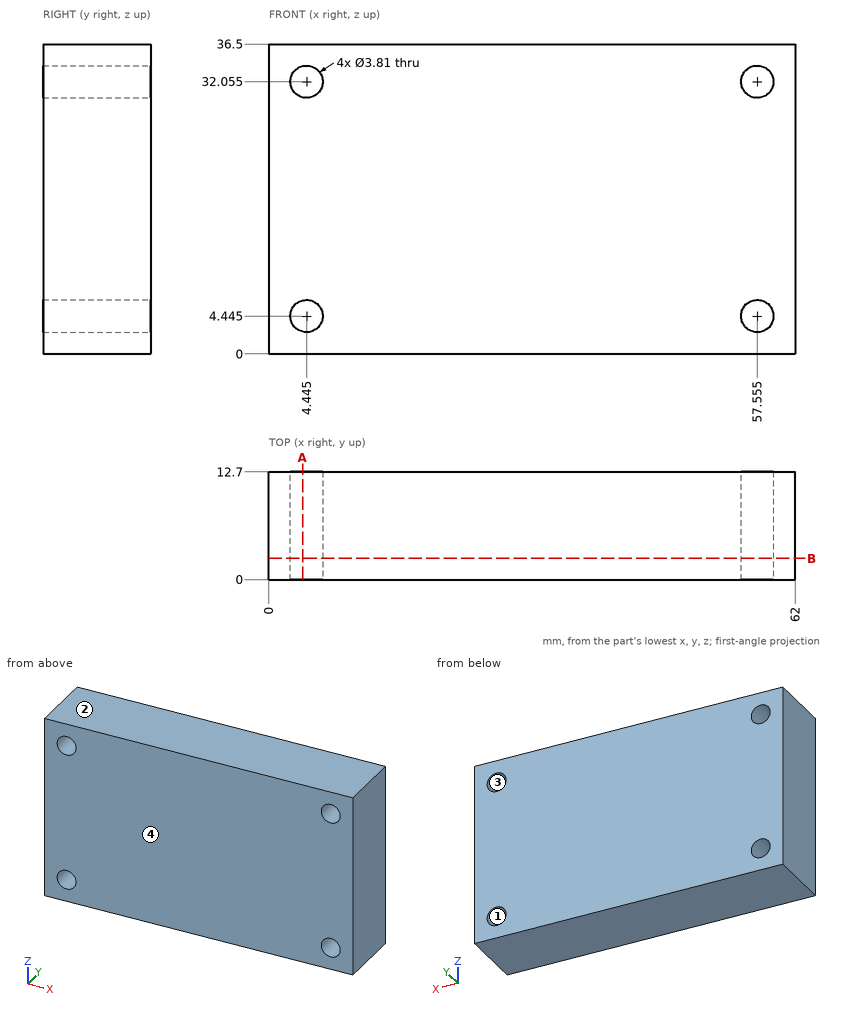
Source: three-view drawing plus pictorial views. Frame: mm from the lowest corner of the part. Coordinates: 2 decimals unless noted, no trailing zeros. Loops run counter-clockwise (first coordinate to the right, second up) from the corner with the lowest first, then second, coordinate; pieces in that order, holes last. Notation, with made-up numbers: (65.25, 46) -> (107.25, 46) arc R23 cw to (107.25, 85) -> close; hole circle Ø11 at (18.25, 52.5). An arc over 180 degrees is marked (long way). One line per item, written item: value.
(1) Cut plane B-B (y = 2.5). Output: boundary loops of the cut face in (x, z) (3 decimals), then the cut area to 3 significant figures.
Answer below:
outline: (0, 0) -> (62, 0) -> (62, 36.5) -> (0, 36.5) -> close; hole circle Ø3.81 at (4.445, 4.445); hole circle Ø3.81 at (4.445, 32.055); hole circle Ø3.81 at (57.555, 4.445); hole circle Ø3.81 at (57.555, 32.055)
area: 2,220 mm2
(2) Draft query along Z for the marked faces 1, 2, 3 and 4. Return one class per face: pulls with the +Z half, pulls with the -Z half, needs draft (parallel to the pull), parting line crosses it, or undercut.
Answer below:
face 1: undercut
face 2: pulls with the +Z half
face 3: undercut
face 4: needs draft
(3) Cut plane A-A (x = 4). Output: boundary loops of the cut face in (y, z).
Answer below:
outline: (0, 0) -> (12.7, 0) -> (12.7, 2.59) -> (0, 2.59) -> close; (0, 6.3) -> (12.7, 6.3) -> (12.7, 30.2) -> (0, 30.2) -> close; (0, 33.91) -> (12.7, 33.91) -> (12.7, 36.5) -> (0, 36.5) -> close
(4) Pin query (flat end, axial travel): pin 1 Ø3 at (x, z) = (4.445, 32.055) entering from +Y. Return the tip coordinate at first contact, or that it passes through.
Answer below:
pin 1: passes through
(5) Ray query, line 1 along Z through (x, y) = (3, 11.25); line 2 along X through (y, z) = (11.25, 33.5); line 3 along X through (y, z) = (8.5, 32.5). Return the intervals inside material, ascending.
Answer below:
line 1: z = 0 to 3.2, 5.69 to 30.81, 33.3 to 36.5
line 2: x = 0 to 3.2, 5.69 to 56.31, 58.8 to 62
line 3: x = 0 to 2.59, 6.3 to 55.7, 59.41 to 62
